Input: dimensioned drawing with shaded views. Units: mm. Origin: part minimum x, y, z. A direction names the side the tool comes from. Round coordinates to 2 decimals unless told otherwise and drop trailing zeros. Loops run counter-clockwise (first coordinate to the right, second up) from the corner with the lowest first, then second, coordinate; pieces in that order, holes last. Notation, with made-up numbers: M 1,-2.75 L 9,-2.75 A8 ccw 9,6.25 Z; hole C 71,-33 d1. An arc over 180 degrees is marked long. Use one line per item in the form item = value. Start each with the question number.
Q1. Section query D-D, the plane z = 14.5. Output: boundary loops of the cut face in (x, y).
Q2. Section query B-B, the plane z = 10. Output: boundary loops of the cut face in (x, y), and give its area (3 significant figures).
Q3. First-contact query: P1, Ø6, axis at x = 15, z = 11.5, coming from the +Y side; P2, Ø6, axis at y = 5.5, z = 2.5, coming from the +X side. Flat tips, straight axial feed; report the tip coordinate or a pass-through.
Q4. Ray query, line 1 along X through (y, z) = (0.6, 10); line 2 along X through (y, z) = (5, 11.75). Return the intervals inside material, ascending.
Q5. Section query A-A, the plane y = 13.5. Output: boundary loops of the cut face in (x, z), and give its area (3 significant figures).
Q6. Access query for the marked faces 1 and 2. Directions: +Z, -Z, +X, -X, +Y, -Y. A direction counts if a zero-diameter tool reaches every point of the face in a straight line with its end or side. Return the directions, or none.
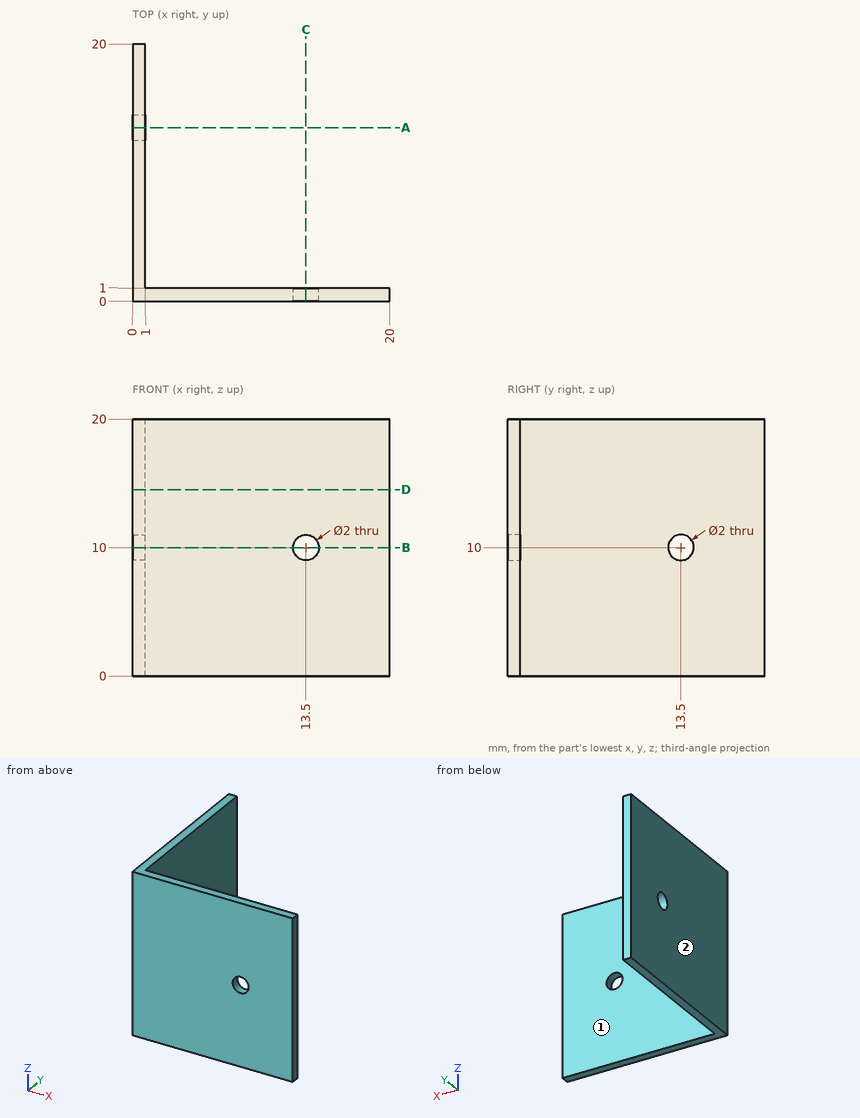
Results found:
q1.outline = M 0,0 L 20,0 L 20,1 L 1,1 L 1,20 L 0,20 Z
q2.outline = M 0,0 L 12.5,0 L 12.5,1 L 1,1 L 1,12.5 L 0,12.5 Z; M 0,14.5 L 1,14.5 L 1,20 L 0,20 Z; M 14.5,0 L 20,0 L 20,1 L 14.5,1 Z
q2.area = 35.0 mm²
q3.P1 = 1
q3.P2 = 1
q4.line_1 = 0 to 12.5, 14.5 to 20
q4.line_2 = 0 to 1
q5.outline = M 0,0 L 1,0 L 1,9 L 0,9 Z; M 0,11 L 1,11 L 1,20 L 0,20 Z
q5.area = 18.0 mm²
q6.face_1 = +Z, -Z, +X, +Y
q6.face_2 = +Z, -Z, -X, +Y, -Y
